```python
from build123d import *

# Parameters (mm, degrees)
F0_R     = 5
F1_DEPTH = 18
F2_SIZE2 = 1
F2_SIZE  = 1
F4_DEPTH = 3


with BuildPart() as f1:
    # F0 (on Top) → F1 (new body)
    with BuildSketch(Plane.XY):
        Circle(F0_R)
    extrude(amount=F1_DEPTH)

    # F2
    f2_edges = [f1.edges().sort_by_distance(p)[0] for p in [
        (-5, 0, 0),
    ]]
    chamfer(f2_edges, length=F2_SIZE, length2=F2_SIZE2)

    # F3 (on face) → F4 (join)
    with BuildSketch(Plane.XY.offset(18)):
        Polygon((8.082904, 0), (4.041452, 7), (-4.041452, 7), (-8.082904, 0), (-4.041452, -7), (4.041452, -7), align=None)
    extrude(amount=F4_DEPTH)


solid = f1.part
```
Part model, mm, in its own coordinate system. A direction names the side the tool comes from. Coordinates: 2 decimals unless noted, no trailing zeros. Write each loop counter-clockwise with the first axis right and the second up, starting at its lowest first coordinate (ties: lowest second). Pieces come first, ordered by that corner, then holes.
Item 1: Probe line 1 (Z direction, x = -7, y = -1.5); line 2 (Y direction, x = 4.5, z = 18.75); line 3 (X direction, y = 1.75, z = 16). List the from-to ranges inside material, lowest first.
Item 2: Slice it at B-B (x = 0). Write the cut outline in (y, z), and give its area (3 significant figures).
Item 3: Pin check, flat tips, straight feed: pin 1 (8 mm diameter, centred on x = 2.5, z = 6.5, fed in from -Y); pin 2 (2 mm diameter, centred on y = 3.5, z = 17.5, fed in from -X); pin 3 (1 mm diameter, centred on x = -4.5, z = 6, fed in from +Y). Stop position of each tip, or through.
Item 4: Slice it at C-C (z = 6.5). Write the cut outline in (x, y).
Item 5: Slice it at A-A (z = 18.5). Write the cut outline in (x, y).
Item 6: Which spindle directions (+Z, -Z, +X, -X, +Y, -Y) get a long thin tool onto all of the face, cutting with end or side? Do faces 1 (the face through (-6.09, -3.45, 19.48)), 2 (the face through (-1.08, -4.88, 9.38)). Say none if no direction does.
Results found:
1. line 1: z = 18 to 21
1. line 2: y = -6.21 to 6.21
1. line 3: x = -4.68 to 4.68
2. outline: (-7, 18) - (-5, 18) - (-5, 1) - (-4, 0) - (4, 0) - (5, 1) - (5, 18) - (7, 18) - (7, 21) - (-7, 21) - close
2. area: 221 mm2
3. pin 1: stops at y = -5
3. pin 2: stops at x = -6.56
3. pin 3: stops at y = 3
4. outline: circle Ø10 at (0, 0)
5. outline: (-8.08, 0) - (-4.04, -7) - (4.04, -7) - (8.08, 0) - (4.04, 7) - (-4.04, 7) - close
6. face 1: +Z, -Z, -X, -Y
6. face 2: -Z
